from build123d import *

# Parameters (mm, degrees)
BOSS_EXTRUDE1_DEPTH = 2


with BuildPart() as part:
    # Sketch1 → Boss-Extrude1 (new body)
    with BuildSketch(Plane(origin=(0, 0, 0), x_dir=(1, 0, 0), z_dir=(0, 1, 0))):
        Polygon((-127, -143), (127, -143), (127, -18), (117, -18), (117, 18), (127, 18), (127, 143), (-127, 143), align=None)
        Polygon((37, 123), (111, 123), (111, 41), (114, 41), (114, -41), (111, -41), (111, -123), (37, -123), (37, -126), (-37, -126), (-37, -123), (-111, -123), (-111, -41), (-114, -41), (-114, 41), (-111, 41), (-111, 123), (-37, 123), (-37, 126), (37, 126), align=None, mode=Mode.SUBTRACT)
    extrude(amount=BOSS_EXTRUDE1_DEPTH)


solid = part.part
Geometry check sheet. Reference: the model listing, model coordinates, mm. Round coordinates to 2 decimals unless told otherwise and drop trailing zeros. Order: outer loops, then holes, each group sorted by start corner. A loop starts at its lowest first (then second) coordinate and runs counter-clockwise, first axis right, second up. Notation, with made-up numbers: M 52.25,12 L 98.25,12 A5 ccw 98.25,19 Z; hole C 9,35 d7. An arc over 180 degrees is marked long. Answer in a Markdown table with one row per item.
(1) Scan lines: probe 1 along X at (y, z) = (0.65, 13); probe 2 along Z at (x, y) = (46, 1.85); probe 3 along Z at (x, y) = (-35, 0.55). Record each from-to range of solid material in increasing order. Write a range as from..to.
Responses:
| item | result |
|---|---|
| probe 1 | x = -127..-114, 114..117 |
| probe 2 | z = -143..-123, 123..143 |
| probe 3 | z = -143..-126, 126..143 |
(2) Sectioned sample at C-C, the plane y = 1.2. Record the cut outline in (x, z).
Responses:
| item | result |
|---|---|
| outline | M -127,-143 L 127,-143 L 127,-18 L 117,-18 L 117,18 L 127,18 L 127,143 L -127,143 Z; hole M -114,-41 L -111,-41 L -111,-123 L -37,-123 L -37,-126 L 37,-126 L 37,-123 L 111,-123 L 111,-41 L 114,-41 L 114,41 L 111,41 L 111,123 L 37,123 L 37,126 L -37,126 L -37,123 L -111,123 L -111,41 L -114,41 Z |
(3) Sectioned sample at B-B, the plane x = -30. Record the cut outline in (y, z), and give its area (3 significant figures).
Responses:
| item | result |
|---|---|
| outline | M 0,-143 L 2,-143 L 2,-126 L 0,-126 Z; M 0,126 L 2,126 L 2,143 L 0,143 Z |
| area | 68.0 mm² |
(4) Sectioned sample at A-A, the plane z = 33.5. Record the cut outline in (x, y), and give its area (3 significant figures).
Responses:
| item | result |
|---|---|
| outline | M -127,0 L -114,0 L -114,2 L -127,2 Z; M 114,0 L 127,0 L 127,2 L 114,2 Z |
| area | 52.0 mm² |
